Could you check a few things on this drawing? It's one solid part, dimensions in mm from its lowest x, y, z. A direction names the side the tool comes from. Give positions to 0.01 mm unless a question says otherwise; leave off trailing zeros. Loops run counter-clockwise (first coordinate to the right, second up) from the corner with the lowest first, then second, coordinate; pieces in that order, holes last. Notation, with made-up numbers: (24.25, 50) -> (65.25, 50) arc R24 cw to (65.25, 73) -> close; hole circle Ø3 at (67.5, 67). An arc over 180 degrees is marked (long way). One line per question, with ' | ' between items.
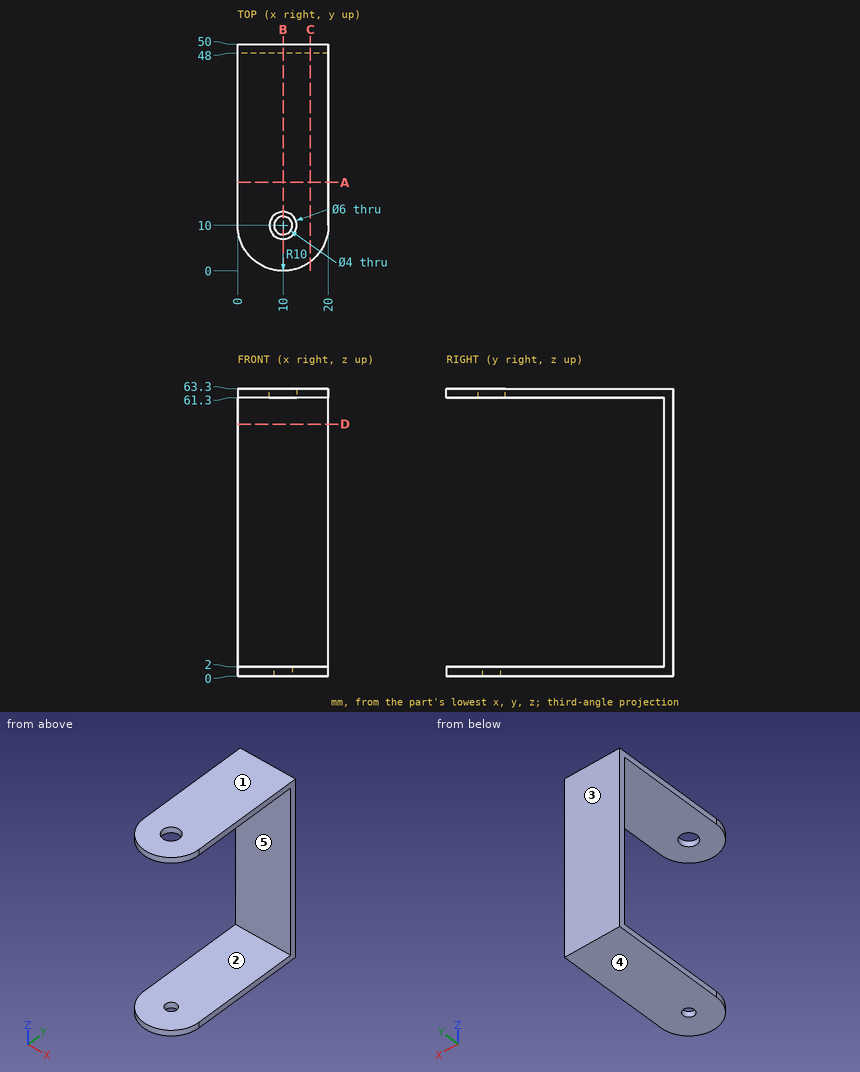
Q1. For pin 1 Ø1.5 at (x, z) = (5, 49.5) entering from -Y, with a flat end and sliding along its axis, tell me the tip position at first contact or that it passes through.
Entries:
pin 1: y = 48
Q2. If we section it at D-D (z = 55.5): Write out the boundary of the cut face in (x, y).
Entries:
outline: (0, 48) -> (20, 48) -> (20, 50) -> (0, 50) -> close
Q3. If I drill on probe 1 along Z at (x, y) = (14.25, 40.5); probe 2 along Y at (x, z) = (10, 0.5); probe 3 along Y at (x, z) = (10, 62.4), over which ranges is the centre line in solid material (lowest first)? Write a range as from..to.
Entries:
probe 1: 0..2, 61.3..63.3 | probe 2: 0..8, 12..50 | probe 3: 0..7, 13..50
Q4. If we section it at B-B (x = 10): Write out the boundary of the cut face in (y, z), plus the area to 3 significant figures.
Entries:
outline: (0, 0) -> (8, 0) -> (8, 2) -> (0, 2) -> close; (0, 61.3) -> (7, 61.3) -> (7, 63.3) -> (0, 63.3) -> close; (12, 0) -> (50, 0) -> (50, 63.3) -> (13, 63.3) -> (13, 61.3) -> (48, 61.3) -> (48, 2) -> (12, 2) -> close | area: 299 mm²
Q5. If we section it at A-A (y = 19.5): Write out the boundary of the cut face in (x, z), plus the area to 3 significant figures.
Entries:
outline: (0, 0) -> (20, 0) -> (20, 2) -> (0, 2) -> close; (0, 61.3) -> (20, 61.3) -> (20, 63.3) -> (0, 63.3) -> close | area: 80.0 mm²
Q6. If we section it at C-C (x = 16): Write out the boundary of the cut face in (y, z), plus the area to 3 significant figures.
Entries:
outline: (2, 0) -> (50, 0) -> (50, 63.3) -> (2, 63.3) -> (2, 61.3) -> (48, 61.3) -> (48, 2) -> (2, 2) -> close | area: 311 mm²
Q7. On a 3-axis mill with a long thin cutter (end or side, diameter ignored), from which of +Z, -Z, +X, -X, +Y, -Y can I reach the whole of each face in a straight line? I mean the marked faces 1 and 2. Say none if no direction works.
Entries:
face 1: +Z, +X, -X, +Y, -Y | face 2: +X, -X, -Y
Q8. If we mould it in two halves opening along Z, with no side actions, what happens to the marked faces 3, 4 and 5? For each: pulls with the +Z half, pulls with the -Z half, needs draft (parallel to the pull), parting line crosses it, or undercut.
Entries:
face 3: needs draft | face 4: pulls with the -Z half | face 5: undercut
